CAD build for the part. Positions are in the model's coordinates, mm. A direction names the side the tool comes from. Give positions to 0.01 mm unless a question says otherwise; leave off trailing zeros. Loops run counter-clockwise (first coordinate to the right, second up) from the corner with the lowest first, then second, coordinate; pieces in that order, holes last.
Autodesk Fusion 360 part; units mm, degrees
sketch "Sketch1" plane through (0, 0, 0) normal (0, 0, 1) x (1, 0, 0)
  line L0 (0, 0) -> (18, 0)
  line L1 (18, 0) -> (18, 21)
  line L2 (18, 21) -> (0, 21)
  line L3 (0, 21) -> (0, 0)
  line L4 (0, 21) -> (35, 21)
  line L5 (35, 21) -> (35, 43)
  line L6 (35, 43) -> (0, 43)
  line L7 (0, 43) -> (0, 21)
  dimension "d1" = 18
  dimension "d2" = 21
  dimension "d18" = 22
extrude "Extrude1" add sketch "Sketch1" along normal blind 3
sketch "Sketch2" plane through (0, 0, 3) normal (0, 0, 1) x (-1, 0, 0)
  line L0 (0, -43) -> (0, 0)
  line L1 (0, 0) -> (-18, 0)
  line L2 (-18, 0) -> (-18, -21)
  line L3 (-18, -21) -> (-35, -21)
  line L4 (-35, -21) -> (-35, -43)
  line L5 (-35, -43) -> (0, -43)
  line L6 (0, -43) -> (-35, -43)
  line L7 (-35, -43) -> (-35, -40)
  line L8 (-35, -40) -> (0, -40)
  line L9 (0, -40) -> (0, -43)
  dimension "d5" = 3
extrude "Extrude2" add sketch "Sketch2" along normal blind 25 contours L0 L4 L5 L6 L7 L8 L9
sketch "Sketch3" plane through (0, 0, 3) normal (0, 0, 1) x (-1, 0, 0)
  line L0 (-35, -40) -> (0, -40)
  line L1 (0, -40) -> (0, 0)
  line L2 (0, 0) -> (-18, 0)
  line L3 (-18, 0) -> (-18, -21)
  line L4 (-18, -21) -> (-35, -21)
  line L5 (-35, -21) -> (-35, -40)
  circle A0 centre (-2, -2) radius 1.5
  circle A1 centre (-2, -20) radius 1.5
  dimension "d8" = 3
  dimension "d9" = 3
extrude "Extrude3" cut sketch "Sketch3" against normal blind 4 contours A0 | A1
sketch "Sketch4" plane through (0, 43, 0) normal (0, 1, 0) x (-1, 0, 0)
  line L0 (-35, 0) -> (0, 0)
  line L1 (0, 0) -> (0, 28)
  line L2 (0, 28) -> (-35, 28)
  line L3 (-35, 28) -> (-35, 0)
  circle A0 centre (-32, 25) radius 1.5
  circle A1 centre (-3, 25) radius 1.5
  circle A2 centre (-3, 7) radius 1.5
  circle A3 centre (-32, 7) radius 1.5
  dimension "d12" = 3
  dimension "d13" = 3
  dimension "d14" = 3
  dimension "d15" = 3
extrude "Extrude4" cut sketch "Sketch4" against normal blind 4 contours A0 | A1 | A2 | A3
thread "Thread1"
thread "Thread2"
thread "Thread3"
thread "Thread4"
thread "Thread5"
thread "Thread6"
1. Saw through at A-A, the plane y = 20. List the corners of the cut face in (x, z), and give its area (3 significant figures).
Responses:
outline: (0, 0) - (0.5, 0) - (0.5, 3) - (0, 3) - close; (3.5, 0) - (18, 0) - (18, 3) - (3.5, 3) - close
area: 45.0 mm2
2. Saw through at C-C, the plane z = 7. List the corners of the cut face in (x, y), and give its area (3 significant figures).
Responses:
outline: (0, 40) - (1.5, 40) - (1.5, 43) - (0, 43) - close; (4.5, 40) - (30.5, 40) - (30.5, 43) - (4.5, 43) - close; (33.5, 40) - (35, 40) - (35, 43) - (33.5, 43) - close
area: 87.0 mm2
3. Probe line 1 along Z through (x, y) = (3, 42); line 2 along Y through (x, z) = (2, 0.7); line 3 along X through (y, z) = (20, 2.4). List the from-to ranges inside material, lowest first.
Responses:
line 1: z = 0 to 5.5, 8.5 to 23.5, 26.5 to 28
line 2: y = 0 to 0.5, 3.5 to 18.5, 21.5 to 43
line 3: x = 0 to 0.5, 3.5 to 18
4. Pull direction Y, two halves, no side cores. Call faces 1 (the face through (13, 27, 0)), 2 (the face through (2.195, 18.513, 1.521)), 3 (the face through (18, 40, 15)): released by +Y, released by -Y, zero draft, split by the parting line, or undercut.
Responses:
face 1: zero draft
face 2: undercut
face 3: released by -Y
5. Drop flat-ended pins along their axis: pin 1 (4 mm diameter, centred on x = 25, z = 11, fed in from -Y); pin 2 (5 mm diameter, centred on x = 32, z = 7, fed in from +Y); pin 3 (5 mm diameter, centred on x = 2, y = 2, fed in from +Z); pin 4 (1.5 mm diameter, centred on y = 6.5, z = 1, fed in from +X). Give the stop position or say it passes through.
Responses:
pin 1: stops at y = 40
pin 2: stops at y = 43
pin 3: stops at z = 3
pin 4: stops at x = 18
6. Saw through at B-B, the plane x = 32. List the corners of the cut face in (y, z).
Responses:
outline: (21, 0) - (43, 0) - (43, 5.5) - (40, 5.5) - (40, 3) - (21, 3) - close; (40, 8.5) - (43, 8.5) - (43, 23.5) - (40, 23.5) - close; (40, 26.5) - (43, 26.5) - (43, 28) - (40, 28) - close
7. Saw through at D-D, the plane x = 3. List the corners of the cut face in (y, z), and give its area (3 significant figures).
Responses:
outline: (0, 0) - (0.88, 0) - (0.88, 3) - (0, 3) - close; (3.12, 0) - (18.88, 0) - (18.88, 3) - (3.12, 3) - close; (21.12, 0) - (43, 0) - (43, 5.5) - (40, 5.5) - (40, 3) - (21.12, 3) - close; (40, 8.5) - (43, 8.5) - (43, 23.5) - (40, 23.5) - close; (40, 26.5) - (43, 26.5) - (43, 28) - (40, 28) - close
area: 173 mm2
8. Tool access for faces 4 (the face through (26, 21, 1)), 5 (the face through (13, 25, 3)), 6 (the face through (35, 41, 9)): list every direction of +Z, -Z, +X, -X, +Y, -Y with a clear straight run to the whole face (end or side of a thin tool).
Responses:
face 4: +Z, -Z, +X, -Y
face 5: +Z, +X, -X, -Y
face 6: +Z, -Z, +X, +Y, -Y
